```python
from build123d import *

# Parameters (mm, degrees)
F1_W     = 50.8
F1_H     = 50.8
F2_DEPTH = 50.8
F3_W     = 50.8
F3_H     = 50.8
F4_DEPTH = 50.8
F5_W     = 50.8
F5_H     = 50.8
F6_DEPTH = 101.6
F7_W     = 50.8
F7_H     = 50.8
F8_DEPTH = 50.8


# Not quite as in the source:
# - a variable given as a bare number and used for a length is read in inches; the dataset says mm whatever the document's units were


with BuildPart() as f2:
    # F1 (on Front) → F2 (new body)
    with BuildSketch(Plane.XZ):
        with Locations((3.1213257462, -3.4399425406)):
            Rectangle(F1_W, F1_H)
    extrude(amount=F2_DEPTH)

    # F3 (on face) → F4 (join)
    with BuildSketch(Plane.XZ.offset(50.8)):
        with Locations((53.9213257462, -3.4399425406)):
            Rectangle(F3_W, F3_H)
    extrude(amount=-F4_DEPTH)

    # F5 (on face) → F6 (join)
    with BuildSketch(Plane.XZ.offset(50.8)):
        with Locations((3.1213257462, -54.2399425406)):
            Rectangle(F5_W, F5_H)
    extrude(amount=-F6_DEPTH)

    # F7 (on face) → F8 (join)
    with BuildSketch(Plane(origin=(0, 50.8, 0), x_dir=(-1, 0, 0), z_dir=(0, 1, 0))):
        with Locations((47.6786742538, -54.2399425406)):
            Rectangle(F7_W, F7_H)
    extrude(amount=-F8_DEPTH)


solid = f2.part
```
Design review of the part built by this model. Coordinates are the model's own, in mm. A direction names the side the tool comes from. Coordinates: 2 decimals unless noted, no trailing zeros. Order: outer loops, then holes, each group sorted by start corner. A loop starts at its lowest first (then second) coordinate and runs counter-clockwise, first axis right, second up. Notation, with made-up numbers: (47.25, -38) -> (101.25, -38) arc R9 ccw to (101.25, -32) -> close; hole circle Ø6 at (-2.5, -21.5). An arc over 180 degrees is marked (long way). One line per item, written item: value. Start each with the question number.
Q1. Take a section at A-A, the plane y = -44. State the section outline as (x, z) points, then the cut area to 3 significant figures.
Q2. Take a section at D-D, the plane x = -26. State the section outline as (y, z) points.
Q3. Take a section at B-B, the plane x = 16. State the section outline as (y, z) points, then the cut area to 3 significant figures.
Q4. Take a section at C-C, the plane z = -21. State the section outline as (x, y) points.
Q5. Tool access review of faces 1 (the flat face through (54, -26, -28.84)), 2 (the flat face through (-22.279, -26, -30)), 3 (the flat face through (-22, 26, -28.84)), 4 (the flat face through (79.321, -26, -4)), 5 (the flat face through (-10, 12, -79.64)): name each direction out of +Z, -Z, +X, -X, +Y, -Y from which nothing blocks a thin tool from reaching the whole face with its end or side.
Q6. Insertion check: pin 1 Ø5 at (x, z) = (39, 9) entering from +Y; pin 2 Ø2 at (x, y) = (44, -31) entering from -Z; pin 3 Ø15 at (y, z) = (-33, -7) entering from -X. Each pin has a flat end and moves straight along its axis. Give the tip position at first contact, or say it passes through.
Q7. For probe 1 along X at (y, z) = (-35, 13); probe 2 along X at (y, z) = (41, -73); probe 3 along Z at (x, y) = (66.5, -42), list the stretches that pass through material, from the lowest coordinate up.
Values follow:
1. outline: (-22.28, -79.64) -> (28.52, -79.64) -> (28.52, -28.84) -> (79.32, -28.84) -> (79.32, 21.96) -> (-22.28, 21.96) -> close
1. area: 7,740 mm2
2. outline: (0, -79.64) -> (50.8, -79.64) -> (50.8, -28.84) -> (0, -28.84) -> close
3. outline: (-50.8, -79.64) -> (50.8, -79.64) -> (50.8, -28.84) -> (0, -28.84) -> (0, 21.96) -> (-50.8, 21.96) -> close
3. area: 7,740 mm2
4. outline: (-22.28, -50.8) -> (79.32, -50.8) -> (79.32, 0) -> (-22.28, 0) -> close
5. face 1: -Z, +X, +Y, -Y
5. face 2: +Z, -Z, -X, -Y
5. face 3: +Z, +X, -X, +Y
5. face 4: +Z, -Z, +X, +Y, -Y
5. face 5: -Z, +X, -X, +Y, -Y
6. pin 1: stops at y = 0
6. pin 2: stops at z = -28.84
6. pin 3: stops at x = -22.28
7. probe 1: x = -22.28 to 79.32
7. probe 2: x = -73.08 to 28.52
7. probe 3: z = -28.84 to 21.96
